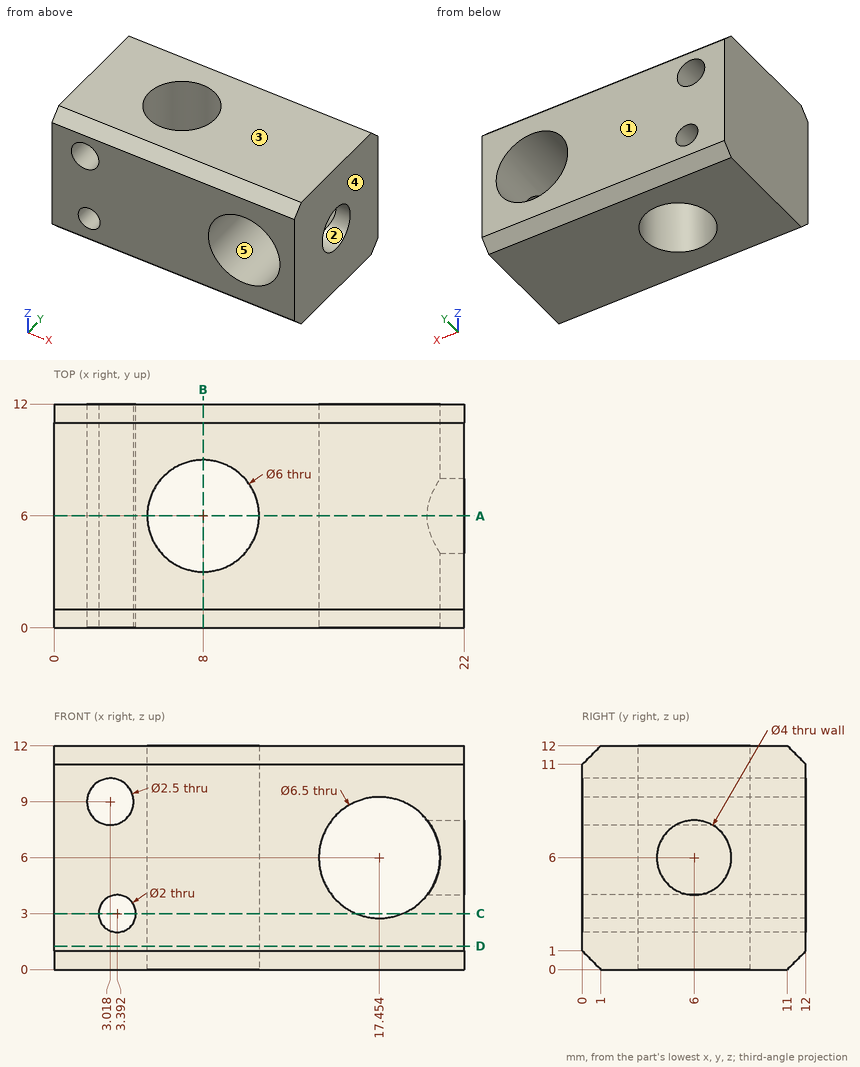
Part print with two shaded views. Sizes in mm from the minimum x, y, z corner. A direction names the side the tool comes from. Coordinates: 2 decimals unless noted, no trailing zeros. Loops run counter-clockwise (first coordinate to the right, second up) from the corner with the lowest first, then second, coordinate; pieces in that order, holes last. Notation, with made-up numbers: (58.5, 72) - (107.5, 72) arc R10 cw to (107.5, 82) - close; hole circle Ø7 at (47, 57.5). An arc over 180 degrees is marked (long way). Write each question's results on one line, items separated by ' | '. Start each with the question number.
Q1. Slice it at A-A on y = 6. Give the number of separate pieces and of enclosed holes in the cut face, and give its area (3 significant figures).
Q2. Probe line 1 along Y through (x, z) = (21.25, 6); line 2 along Z through (x, y) = (3, 6); line 3 along X through (y, z) = (3.5, 3.25) (1 decimal). List the from-to ranges inside material, lowest first.
Q3. Slice it at C-C on z = 3. Give the cut face in (x, y) (1 decimal), and give its area (3 significant figures).
Q4. Slice it at D-D on z = 1.25. Give the cut face in (x, y).
Q5. Which spindle directions (+Z, -Z, +X, -X, +Y, -Y) get a long thin tool onto all of the face, cutting with end or side? Do the marked faces 1 and 2. Say none if no direction does.
Q6. Two-plate mould, pull along Z, no slides. Class the marked faces 3, 4 and 5: +Z half, -Z half, draft (parallel to the pull), parting line (faces both ways), or undercut.
Q7. Slice it at B-B on x = 8. Give the cut face in (y, z), and give its area (3 significant figures).
Q8. Drop a flat-ended pin along its axis: pin 1 Ø2.5 at (x, z) = (3.39, 3) entering from -Y. Give the stop position or say it passes through.
Answer:
1) separate pieces: 2 | enclosed holes: 2 | area: 145 mm2
2) line 1: y = 0 to 4, 8 to 12 | line 2: z = 0 to 2.08, 3.92 to 7.75, 10.25 to 12 | line 3: x = 0 to 2.4, 4.4 to 6.3, 9.7 to 15.7, 19.2 to 22
3) outline: (0, 0) - (2.4, 0) - (2.4, 12) - (0, 12) - close; (4.4, 0) - (16.2, 0) - (16.2, 12) - (4.4, 12) - close; (18.7, 0) - (22, 0) - (22, 12) - (18.7, 12) - close; hole circle Ø6 at (8, 6) | area: 182 mm2
4) outline: (0, 0) - (22, 0) - (22, 12) - (0, 12) - close; hole circle Ø6 at (8, 6)
5) face 1: +Z, -Z, +X, -X, +Y | face 2: +X
6) face 3: +Z half | face 4: draft | face 5: undercut
7) outline: (0, 1) - (1, 0) - (3, 0) - (3, 12) - (1, 12) - (0, 11) - close; (9, 0) - (11, 0) - (12, 1) - (12, 11) - (11, 12) - (9, 12) - close | area: 70.0 mm2
8) pin 1: stops at y = 0
